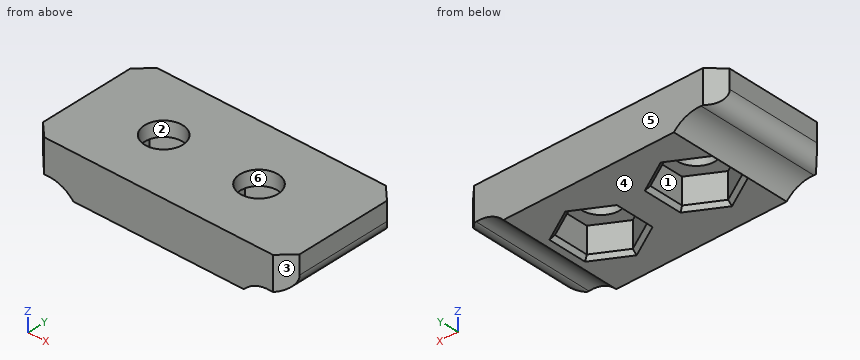
```python
from build123d import *

# Parameters (mm, degrees)
SKETCH1_W           = 35
SKETCH1_H           = 21
BOSS_EXTRUDE1_DEPTH = 6
SKETCH2_W           = 35
SKETCH2_H           = 21
SKETCH2_R           = 2.6
BOSS_EXTRUDE2_DEPTH = 2
CHAMFER1_SIZE       = 4
CHAMFER2_SIZE       = 0.5
SKETCH3_R           = 4.499999999
SKETCH3_R_2         = 4.500000001
CUT_EXTRUDE1_DEPTH  = 49.5
FILLET1_R           = 2
FILLET2_R           = 2
SKETCH5_W           = 39.219322143
SKETCH5_H           = 6.192524549
SKETCH5_W_2         = 37.895134504
SKETCH5_H_2         = 8.100912618
CUT_EXTRUDE2_DEPTH  = 10


with BuildPart() as part:
    # Sketch1 → Boss-Extrude1 (new body)
    with BuildSketch(Plane(origin=(0, 0, 789.620141885), x_dir=(-1, 0, 0), z_dir=(0, 0, -1))):
        with Locations((-45.789156386, -208.298939869)):
            Rectangle(SKETCH1_W, SKETCH1_H)
        Polygon((-51.789156386, -203.564667662), (-55.889156386, -205.931803766), (-55.889156386, -210.666075973), (-51.789156386, -213.033212077), (-47.689156386, -210.666075973), (-47.689156386, -205.931803766), align=None, mode=Mode.SUBTRACT)
        Polygon((-42.889156386, -205.931803766), (-42.889156386, -210.666075973), (-38.789156386, -213.033212077), (-34.689156386, -210.666075973), (-34.689156386, -205.931803766), (-38.789156386, -203.564667662), align=None, mode=Mode.SUBTRACT)
    extrude(amount=BOSS_EXTRUDE1_DEPTH)

    # Sketch2 → Boss-Extrude2 (add)
    with BuildSketch(Plane.XY.offset(789.620141885)):
        with Locations((45.789156386, -208.298939869)):
            Rectangle(SKETCH2_W, SKETCH2_H)
        with Locations((38.789156386, -208.298939869)):
            Circle(SKETCH2_R, mode=Mode.SUBTRACT)
        with Locations((51.789156386, -208.298939869)):
            Circle(SKETCH2_R, mode=Mode.SUBTRACT)
    extrude(amount=-BOSS_EXTRUDE2_DEPTH)

    # Chamfer1
    chamfer1_edges = [part.edges().sort_by_distance(p)[0] for p in [
        (63.289156386, -197.798939869, 786.620141885),
        (28.289156386, -197.798939869, 786.620141885),
        (28.289156386, -218.798939869, 786.620141885),
        (63.289156386, -218.798939869, 786.620141885),
    ]]
    chamfer(chamfer1_edges, length=CHAMFER1_SIZE)

    # Chamfer2
    chamfer2_edges = [part.edges().sort_by_distance(p)[0] for p in [
        (45.789156386, -197.798939869, 783.620141885),
        (45.789156386, -218.798939869, 783.620141885),
        (28.289156386, -208.298939869, 783.620141885),
        (61.289156386, -216.798939869, 783.620141885),
        (30.289156386, -216.798939869, 783.620141885),
        (30.289156386, -199.798939869, 783.620141885),
        (61.289156386, -199.798939869, 783.620141885),
        (49.739156386, -204.748235714, 783.620141885),
        (53.839156386, -204.748235714, 783.620141885),
        (55.889156386, -208.298939869, 783.620141885),
        (53.839156386, -211.849644025, 783.620141885),
        (49.739156386, -211.849644025, 783.620141885),
        (47.689156386, -208.298939869, 783.620141885),
        (40.839156386, -204.748235714, 783.620141885),
        (42.889156386, -208.298939869, 783.620141885),
        (40.839156386, -211.849644025, 783.620141885),
        (36.739156386, -211.849644025, 783.620141885),
        (34.689156386, -208.298939869, 783.620141885),
        (36.739156386, -204.748235714, 783.620141885),
        (63.289156386, -208.298939869, 783.620141885),
    ]]
    chamfer(chamfer2_edges, length=CHAMFER2_SIZE)

    # Sketch3 → Cut-Extrude1 (cut)
    with BuildSketch(Plane(origin=(0, -197.798939869, 0), x_dir=(1, 0, 0), z_dir=(0, 1, 0))):
        with Locations((30.822197264, -780.620141885)):
            Circle(SKETCH3_R)
        with Locations((60.756115509, -780.620141885)):
            Circle(SKETCH3_R_2)
    extrude(amount=-CUT_EXTRUDE1_DEPTH, mode=Mode.SUBTRACT)

    # Fillet1
    fillet1_edges = [part.edges().sort_by_distance(p)[0] for p in [
        (28.289156386, -208.298939869, 784.339510636),
    ]]
    fillet(fillet1_edges, radius=FILLET1_R)

    # Fillet2
    fillet2_edges = [part.edges().sort_by_distance(p)[0] for p in [
        (63.289156386, -208.298939869, 784.339510637),
    ]]
    fillet(fillet2_edges, radius=FILLET2_R)

    # Sketch5 → Cut-Extrude2 (cut)
    with BuildSketch(Plane(origin=(0, 0, 783.620141885), x_dir=(-1, 0, 0), z_dir=(0, 0, -1))):
        with Locations((-46.0812566, -196.802677595)):
            Rectangle(SKETCH5_W, SKETCH5_H)
        with Locations((-45.419162781, -220.749396178)):
            Rectangle(SKETCH5_W_2, SKETCH5_H_2)
    extrude(amount=-CUT_EXTRUDE2_DEPTH, mode=Mode.SUBTRACT)


solid = part.part
```
Design review of the part built by this model. Coordinates are the model's own, in mm. Face numbers are marked on the shaded views. A direction names the side the tool comes from. Round coordinates to 2 decimals unless told otherwise and drop trailing zeros. Order: outer loops, then holes, each group sorted by start corner. A loop starts at its lowest first (then second) coordinate and runs counter-clockwise, first axis right, second up. Notation, with made-up numbers: (48, 49.25) - (70, 49.25) arc R17 cw to (70, 77.25) - close; hole circle Ø11 at (46.5, 14.5). An arc over 180 degrees is marked (long way). One line per question, with ' | ' between items.
Item 1: Wall thickness on line 1 (Y direction, x = 42.5, z = 786); line 2 (X direction, y = -204.25, z = 786.25); line 3 (X direction, y = -208, z = 786.5): over which ranges is each line inside the solid? List them lowest first. Write a range as [from, to].
Checks:
line 1: [-216.7, -210.89], [-205.71, -199.9] | line 2: [28.48, 37.6], [39.98, 50.6], [52.98, 63.1] | line 3: [28.38, 34.69], [42.89, 47.69], [55.89, 63.2]
Item 2: Take a section at D-D, the plane x = 55. Write out the cut boundary in (y, z).
Checks:
outline: (-216.7, 783.62) - (-211.76, 783.62) - (-211.18, 784.12) - (-211.18, 787.62) - (-205.42, 787.62) - (-205.42, 784.12) - (-204.84, 783.62) - (-199.9, 783.62) - (-199.9, 789.62) - (-216.7, 789.62) - close
Item 3: For P1, Ø1.8, axis at y = -208, z = 786, coming from the -X side; P2, Ø3, axis at y = -208.5, z = 785.5, coming from the +X side; P3, Ø6, axis at x = 38.79, y = -208.3, coming from the -Z side, all flat-tipped, find the tip position at first contact; note any pin that passes through.
Checks:
P1: x = 28.3 | P2: x = 63.29 | P3: z = 787.62
Item 4: Draft analysis for pull direction Y (two halves, no side actions). For the marked faces 3, 4, 5 and 6, state which applies: +Y half, -Y half, draft (parallel to the pull), parting line (faces both ways), or undercut.
Checks:
face 3: -Y half | face 4: draft | face 5: +Y half | face 6: undercut
Item 5: Machinability: for the marked faces 1 and 2, which of the approach directions +Z, -Z, +X, -X, +Y, -Y give a long, thin tool a straight path to every point of the face, cutting with its end or side? Answer none if there is none.
Checks:
face 1: -Z | face 2: +Z, -Z
Item 6: Take a section at B-B, the plane x = 50. Write out the cut boundary in (y, z).
Checks:
outline: (-216.7, 783.62) - (-212.58, 783.62) - (-212, 784.12) - (-212, 787.62) - (-210.19, 787.62) - (-210.19, 789.62) - (-216.7, 789.62) - close; (-206.41, 787.62) - (-204.6, 787.62) - (-204.6, 784.12) - (-204.02, 783.62) - (-199.9, 783.62) - (-199.9, 789.62) - (-206.41, 789.62) - close
Item 7: Take a section at A-A, the plane y = -207.5. Give the number of separate pieces and of enclosed holes in the cut face, then the cut area to 3 significant figures.
Checks:
separate pieces: 3 | enclosed holes: 0 | area: 108 mm²
Item 8: Take a section at C-C, the plane z = 788.5. Write out the cut boundary in (x, y).
Checks:
outline: (28.29, -214.8) - (30.19, -216.7) - (61.39, -216.7) - (63.29, -214.8) - (63.29, -201.8) - (61.39, -199.9) - (30.19, -199.9) - (28.29, -201.8) - close; hole circle Ø5.2 at (38.79, -208.3); hole circle Ø5.2 at (51.79, -208.3)
